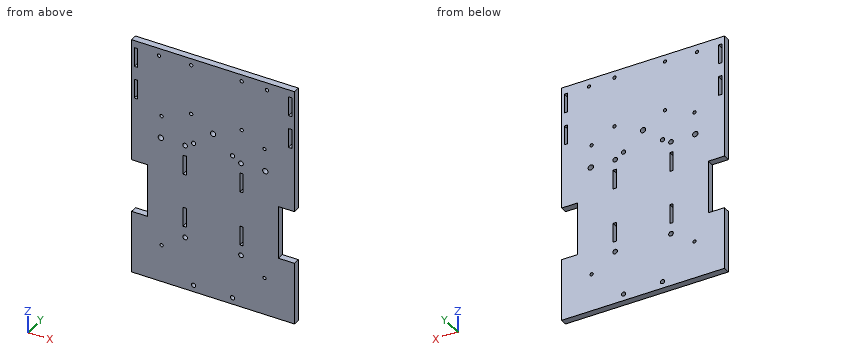
```python
from build123d import *

# Parameters (mm, degrees)
SKETCH2_W           = 154.686
SKETCH2_H           = 228.6
BOSS_EXTRUDE1_DEPTH = 6.35
SKETCH1_R           = 2.2225
CUT_EXTRUDE1_DEPTH  = 6.35
SKETCH3_W           = 15.24
SKETCH3_H           = 50.8
CUT_EXTRUDE2_DEPTH  = 6.35
SKETCH8_R           = 2.54
CUT_EXTRUDE3_DEPTH  = 17.78
SKETCH9_R           = 1.5875
CUT_EXTRUDE4_DEPTH  = 17.78
SKETCH10_R          = 1.5875
CUT_EXTRUDE5_DEPTH  = 10.16
SKETCH12_W          = 3.048
SKETCH12_H          = 18.542
CUT_EXTRUDE7_DEPTH  = 8.255
SKETCH13_W          = 3.2258
SKETCH13_H          = 18.542
CUT_EXTRUDE8_DEPTH  = 7.35
SKETCH14_R          = 1.5875
CUT_EXTRUDE9_DEPTH  = 7.35
SKETCH16_R          = 2
CUT_EXTRUDE11_DEPTH = 7.35


with BuildPart() as part:
    # Sketch2 → Boss-Extrude1 (new body)
    with BuildSketch(Plane(origin=(0, 0, 0), x_dir=(1, 0, 0), z_dir=(0, 1, 0))):
        with Locations((26.543, 26.944051327)):
            Rectangle(SKETCH2_W, SKETCH2_H)
    extrude(amount=BOSS_EXTRUDE1_DEPTH)

    # Sketch1 → Cut-Extrude1 (cut)
    with BuildSketch(Plane(origin=(0, 0, 0), x_dir=(1, 0, 0), z_dir=(0, 1, 0))):
        with Locations((0, 90.444051327)):
            Circle(SKETCH1_R)
        with Locations((53.086, 90.444051327)):
            Circle(SKETCH1_R)
        Circle(SKETCH1_R)
        with Locations((53.086, 0)):
            Circle(SKETCH1_R)
    extrude(amount=CUT_EXTRUDE1_DEPTH, mode=Mode.SUBTRACT)

    # Sketch3 → Cut-Extrude2 (cut)
    with BuildSketch(Plane(origin=(0, 6.35, 0), x_dir=(1, 0, 0), z_dir=(0, 1, 0))):
        with Locations((96.266, 56.154051327)):
            Rectangle(SKETCH3_W, SKETCH3_H)
        with Locations((-43.18, 56.154051327)):
            Rectangle(SKETCH3_W, SKETCH3_H)
    extrude(amount=-CUT_EXTRUDE2_DEPTH, mode=Mode.SUBTRACT)

    # Sketch8 → Cut-Extrude3 (cut)
    with BuildSketch(Plane(origin=(0, 6.35, 0), x_dir=(1, 0, 0), z_dir=(0, 1, 0))):
        with Locations((26.550112, -20.29968)):
            Circle(SKETCH8_R)
        with Locations((-23.077082804, 0.02032)):
            Circle(SKETCH8_R)
        with Locations((76.177306804, 0.02032)):
            Circle(SKETCH8_R)
    extrude(amount=-CUT_EXTRUDE3_DEPTH, mode=Mode.SUBTRACT)

    # Sketch9 → Cut-Extrude4 (cut)
    with BuildSketch(Plane(origin=(0, 6.35, 0), x_dir=(1, 0, 0), z_dir=(0, 1, 0))):
        with Locations((53.722112, -33.005948673)):
            Circle(SKETCH9_R)
        with Locations((5.722112, -33.005948673)):
            Circle(SKETCH9_R)
        with Locations((53.722112, -81.005948673)):
            Circle(SKETCH9_R)
        with Locations((5.722112, -81.005948673)):
            Circle(SKETCH9_R)
    extrude(amount=-CUT_EXTRUDE4_DEPTH, mode=Mode.SUBTRACT)

    # Sketch10 → Cut-Extrude5 (cut)
    with BuildSketch(Plane(origin=(0, 6.35, 0), x_dir=(1, 0, 0), z_dir=(0, 1, 0))):
        with Locations((-22.3266, 105.430051327)):
            Circle(SKETCH10_R)
        with Locations((-22.3266, -21.569948673)):
            Circle(SKETCH10_R)
        with Locations((75.4126, 105.430051327)):
            Circle(SKETCH10_R)
        with Locations((75.4126, -21.569948673)):
            Circle(SKETCH10_R)
    extrude(amount=-CUT_EXTRUDE5_DEPTH, mode=Mode.SUBTRACT)

    # Sketch12 → Cut-Extrude7 (cut)
    with BuildSketch(Plane(origin=(0, 6.35, 0), x_dir=(1, 0, 0), z_dir=(0, 1, 0))):
        with Locations((-0.373888, 19.451051327)):
            Rectangle(SKETCH12_W, SKETCH12_H)
        with Locations((-0.373888, 70.759051327)):
            Rectangle(SKETCH12_W, SKETCH12_H)
        with Locations((53.474112, 71.267051327)):
            Rectangle(SKETCH12_W, SKETCH12_H)
        with Locations((53.474112, 18.943051327)):
            Rectangle(SKETCH12_W, SKETCH12_H)
    extrude(amount=-CUT_EXTRUDE7_DEPTH, mode=Mode.SUBTRACT)

    # Sketch13 → Cut-Extrude8 (cut, through all)
    with BuildSketch(Plane(origin=(0, 6.35, 0), x_dir=(1, 0, 0), z_dir=(0, 1, 0))):
        with Locations((-46.6471, -39.984948673)):
            Rectangle(SKETCH13_W, SKETCH13_H)
        with Locations((-46.6471, -71.226948673)):
            Rectangle(SKETCH13_W, SKETCH13_H)
        with Locations((99.7331, -71.226948673)):
            Rectangle(SKETCH13_W, SKETCH13_H)
        with Locations((99.7331, -39.984948673)):
            Rectangle(SKETCH13_W, SKETCH13_H)
    extrude(amount=-CUT_EXTRUDE8_DEPTH, mode=Mode.SUBTRACT)

    # Sketch14 → Cut-Extrude9 (cut, through all)
    with BuildSketch(Plane(origin=(0, 6.35, 0), x_dir=(1, 0, 0), z_dir=(0, 1, 0))):
        with Locations((-24.765, -80.309322307)):
            Circle(SKETCH14_R)
        with Locations((77.851, -80.309322307)):
            Circle(SKETCH14_R)
    extrude(amount=-CUT_EXTRUDE9_DEPTH, mode=Mode.SUBTRACT)

    # Sketch16 → Cut-Extrude11 (cut, through all)
    with BuildSketch(Plane(origin=(0, 6.35, 0), x_dir=(1, 0, 0), z_dir=(0, 1, 0))):
        with Locations((45.060116, 134.894051327)):
            Circle(SKETCH16_R)
        with Locations((8.040116, 134.894051327)):
            Circle(SKETCH16_R)
        with Locations((8.040116, -4.805948673)):
            Circle(SKETCH16_R)
        with Locations((45.060116, -4.805948673)):
            Circle(SKETCH16_R)
    extrude(amount=-CUT_EXTRUDE11_DEPTH, mode=Mode.SUBTRACT)


solid = part.part
```
Can you work these out from the model? Positions are in its coordinate system, mm. Coordinates: 2 decimals unless noted, no trailing zeros. Loops run counter-clockwise (first coordinate to the right, second up) from the corner with the lowest first, then second, coordinate; pieces in that order, holes last. Notation, with made-up numbers: M 62,-14 L 109,-14 A25 ccw 109,2 Z; hole C 84,21 d1. An arc over 180 degrees is marked long. Put each result on its own line as item: value. Start each with the question number.
(1) Imagine slicing it at A-A on z = 70. List the corners of the cut face in (x, y) for me.
(2) Imagine slicing it at B-B on z = -50.5. List the corners of the cut face in (x, y) for me.
(3) Imagine slicing it at C-C on y = 2. Give the number of separate pieces and of enclosed holes in the cut face, and give its area (3 significant figures).
(4) Will this pin go through, and if not, where does the flat tip stop? pin 1 Ø3 at (x, z) = (26.55, 20.3) entering from -Y.
(5) I need wall thicknesses on probe 1 along X at (y, z) = (6, 36); probe 2 along X at (y, z) = (3.5, 0); probe 3 along Z at (x, y) = (-42, 4). Which ranges of each line are inside material? Lowest first, please.
Worked answers:
1. outline: M -50.8,0 L -48.26,0 L -48.26,6.35 L -50.8,6.35 Z; M -45.03,0 L 98.12,0 L 98.12,6.35 L -45.03,6.35 Z; M 101.35,0 L 103.89,0 L 103.89,6.35 L 101.35,6.35 Z
2. outline: M -35.56,0 L 88.65,0 L 88.65,6.35 L -35.56,6.35 Z
3. separate pieces: 1
3. enclosed holes: 29
3. area: 33,100 mm2
4. pin 1: passes through
5. probe 1: x = -50.8 to -48.26, -45.03 to 98.12, 101.35 to 103.89
5. probe 2: x = -50.8 to -25.62, -20.54 to -2.22, 2.22 to 50.86, 55.31 to 73.64, 78.72 to 103.89
5. probe 3: z = -141.24 to -81.55, -30.75 to 87.36
